The listing builds one solid part. Answer for the finished solid, in the listing's coordinates (mm). Coordinates: 2 decimals unless noted, no trailing zeros. Loops run counter-clockwise (first coordinate to the right, second up) from the corner with the lowest first, then second, coordinate; pieces in that order, holes last. Notation, with made-up numbers: M 49.5,60 L 78.5,60 A14 ccw 78.5,73 Z; hole C -38,-8 d11. An arc over 180 degrees is marked long. Return JSON: item names as keys, results as strings. Group by question number.
1. Section B-B (z = -18.5) is taken. Write down the section's boundary in (x, y), then the cut area to 4 significant figures.
2. Straight lines are drawn through the part: L1, parallel to Z at x = 18, y = 2.9; L2, parallel to Y at x = 4.5, z = -2.75; L3, parallel to X at y = 1.15, z = -6.25. For each, find the intervals that lie inside material, in ascending order. Write a range as from..to.
3. Section D-D (x = 16) is taken. Write down the section's boundary in (y, z).
4. Section A-A (x = 40.5) is taken. Write down the section's boundary in (y, z).
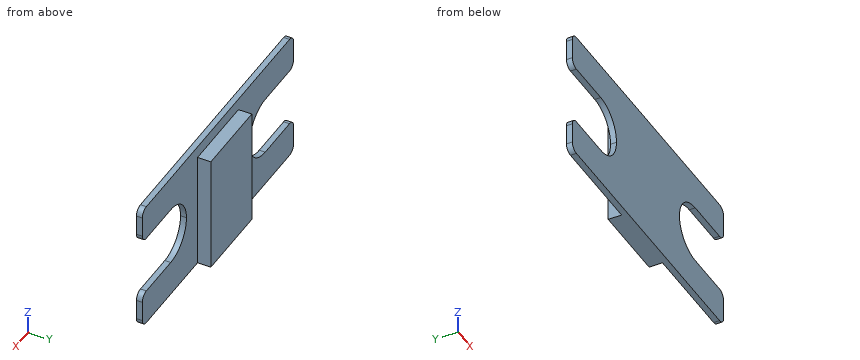
```python
from build123d import *

# Parameters (mm, degrees)
BOSS_EXTRUDE1_DEPTH = 1
FILLET1_R           = 1.27
FILLET2_R           = 5
SKETCH2_W           = 13
SKETCH2_H           = 20
BOSS_EXTRUDE2_DEPTH = 2.25


with BuildPart() as part:
    # Sketch1 → Boss-Extrude1 (new body)
    with BuildSketch(Plane(origin=(0, 0, 0), x_dir=(1, 0, 0), z_dir=(0, 1, 0))):
        Polygon((0, 0), (0, 6), (14, 6), (14, 16), (0, 16), (0, 22), (48, 22), (48, 16), (34, 16), (34, 6), (48, 6), (48, 0), align=None)
    extrude(amount=BOSS_EXTRUDE1_DEPTH)

    # Fillet1
    fillet1_edges = [part.edges().sort_by_distance(p)[0] for p in [
        (0, 0.5, 0),
        (0, 0.5, -6),
        (0, 0.5, -16),
        (0, 0.5, -22),
        (48, 0.5, -22),
        (48, 0.5, -16),
        (48, 0.5, -6),
        (48, 0.5, 0),
    ]]
    fillet(fillet1_edges, radius=FILLET1_R)

    # Fillet2
    fillet2_edges = [part.edges().sort_by_distance(p)[0] for p in [
        (34, 0.5, -6),
        (34, 0.5, -16),
        (14, 0.5, -6),
        (14, 0.5, -16),
    ]]
    fillet(fillet2_edges, radius=FILLET2_R - 0.0001)  # a hair under: the kernel refuses the full size

    # Sketch2 → Boss-Extrude2 (add)
    with BuildSketch(Plane(origin=(0, 1, 0), x_dir=(1, 0, 0), z_dir=(0, 1, 0))):
        with Locations((24, 12)):
            Rectangle(SKETCH2_W, SKETCH2_H)
    extrude(amount=BOSS_EXTRUDE2_DEPTH)


solid = part.part
```
Worked out:
{
 "1": {"outline": "M 0,0 L 48,0 L 48,1 L 30.5,1 L 30.5,3.25 L 17.5,3.25 L 17.5,1 L 0,1 Z", "area": "77.25 mm^2"},
 "2": {"L1": "-22..-2", "L2": "0..1", "L3": "17.5..30.5"},
 "3": {"outline": "M 0,-22 L 1,-22 L 1,0 L 0,0 Z"},
 "4": {"outline": "M 0,-22 L 1,-22 L 1,-16 L 0,-16 Z; M 0,-6 L 1,-6 L 1,0 L 0,0 Z"}
}
